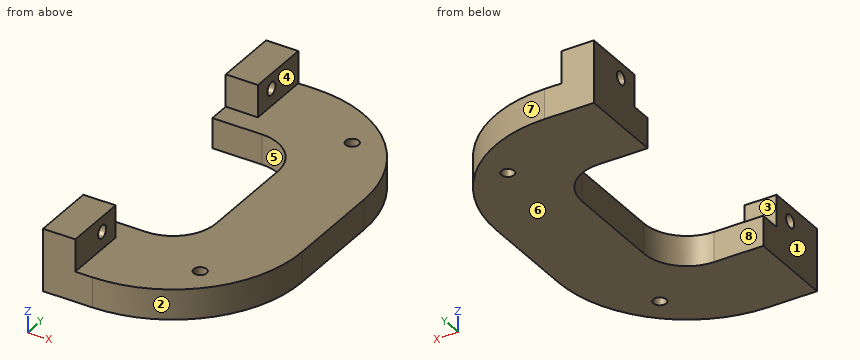
```python
from build123d import *

# Parameters (mm, degrees)
BOSS_EXTRUDE4_DEPTH = 7
SKETCH6_W           = 7.5
SKETCH6_H           = 20
BOSS_EXTRUDE5_DEPTH = 7.5
SKETCH7_R           = 1.5
CUT_EXTRUDE3_DEPTH  = 7.5
SKETCH8_R           = 1.5
CUT_EXTRUDE4_DEPTH  = 7.5
SKETCH9_W           = 7.5
SKETCH9_H           = 5
CUT_EXTRUDE5_DEPTH  = 7.5


with BuildPart() as part:
    # Sketch1 → Boss-Extrude4 (new body)
    with BuildSketch(Plane.XY):
        with BuildLine():
            Line((41.5, -11.5), (41.5, 11.5))
            ThreePointArc((41.5, 11.5), (32.713203436, 32.713203436), (11.5, 41.5))
            Line((11.5, 41.5), (0, 41.5))
            Line((0, 41.5), (0, 21.5))
            Line((0, 21.5), (11.5, 21.5))
            ThreePointArc((11.5, 21.5), (18.571067812, 18.571067812), (21.5, 11.5))
            Line((21.5, 11.5), (21.5, -11.5))
            ThreePointArc((21.5, -11.5), (18.571067812, -18.571067812), (11.5, -21.5))
            Line((11.5, -21.5), (0, -21.5))
            Line((0, -21.5), (0, -41.5))
            Line((0, -41.5), (11.5, -41.5))
            ThreePointArc((11.5, -41.5), (32.713203436, -32.713203436), (41.5, -11.5))
        make_face()
    extrude(amount=BOSS_EXTRUDE4_DEPTH)

    # Sketch6 → Boss-Extrude5 (add)
    with BuildSketch(Plane.XY.offset(7)):
        with Locations((3.75, 31.5)):
            Rectangle(SKETCH6_W, SKETCH6_H)
        with Locations((3.75, -31.5)):
            Rectangle(SKETCH6_W, SKETCH6_H)
    extrude(amount=BOSS_EXTRUDE5_DEPTH)

    # Sketch7 → Cut-Extrude3 (cut)
    with BuildSketch(Plane(origin=(7.5, 0, 0), x_dir=(0, 0, -1), z_dir=(1, 0, 0))):
        with Locations((-11, 31.5)):
            Circle(SKETCH7_R)
        with Locations((-11, -31.5)):
            Circle(SKETCH7_R)
    extrude(amount=-CUT_EXTRUDE3_DEPTH, mode=Mode.SUBTRACT)

    # Sketch8 → Cut-Extrude4 (cut)
    with BuildSketch(Plane.XY.offset(7)):
        with Locations((28.284271247, 28.284271247)):
            Circle(SKETCH8_R)
        with Locations((28.284271247, -28.284271247)):
            Circle(SKETCH8_R)
    extrude(amount=-CUT_EXTRUDE4_DEPTH, mode=Mode.SUBTRACT)

    # Sketch9 → Cut-Extrude5 (cut)
    with BuildSketch(Plane(origin=(7.5, 0, 0), x_dir=(0, 0, -1), z_dir=(1, 0, 0))):
        with Locations((-10.75, 24)):
            Rectangle(SKETCH9_W, SKETCH9_H)
        with Locations((-10.75, -24)):
            Rectangle(SKETCH9_W, SKETCH9_H)
    extrude(amount=-CUT_EXTRUDE5_DEPTH, mode=Mode.SUBTRACT)


solid = part.part
```
Could you check a few things on this model? Use its own coordinates, in mm. Face numbers are marked on the shaded views. A direction names the side the tool comes from. Round coordinates to 2 decimals unless told otherwise and drop trailing zeros. Write each loop counter-clockwise with the first axis right and the second up, starting at its lowest first coordinate (ties: lowest second). Pieces come first, ordered by that corner, then holes.
(1) Suppose I cut it at D-D on x = 37.5. Write out the boundary of the cut face in (y, z).
Findings below:
outline: (-26.47, 0) - (26.47, 0) - (26.47, 7) - (-26.47, 7) - close
(2) Thinking about a two-plate mould opening in Y: for the marked faces 6, 7 and 8, which applies, +Y half, -Y half, draft (parallel to the pull), parting line (faces both ways), or undercut?
Findings below:
face 6: draft
face 7: +Y half
face 8: undercut
(3) Suppose I cut it at A-A on z = 11. Write out the boundary of the cut face in (x, y).
Findings below:
outline: (0, -41.5) - (7.5, -41.5) - (7.5, -33) - (0, -33) - close; (0, -30) - (7.5, -30) - (7.5, -26.5) - (0, -26.5) - close; (0, 26.5) - (7.5, 26.5) - (7.5, 30) - (0, 30) - close; (0, 33) - (7.5, 33) - (7.5, 41.5) - (0, 41.5) - close
(4) For pin 1 (4 mm diameter, centred on y = -31.5, z = 11, fed in from -X); pin 2 (3.5 mm diameter, centred on y = -3.5, z = 4, fed in from -X); pin 3 (2 mm diameter, centred on y = 35.5, z = 11.5, fed in from +X); pin 4 (4 mm diameter, centred on x = 19, z = 6.5, fed in from -Y), each with a flat end and sliding along its axis, tell me the tip position at first contact or that it passes through.
Findings below:
pin 1: stops at x = 0
pin 2: stops at x = 21.5
pin 3: stops at x = 7.5
pin 4: stops at y = -40.99
(5) Which directions (+Z, -Z, +X, -X, +Y, -Y) give clear straight access to the entire face, cutting with the end or side of a thin tool? Please do the marked faces 1, 2, 3, 4 and 5.
Findings below:
face 1: +Z, -Z, -X, +Y, -Y
face 2: +Z, -Z, +X, -Y
face 3: +Z, +X, -X
face 4: +Z, +X, +Y, -Y
face 5: +Z, -Z, -X
(6) If I drill on probe 1 along Y at (x, z) = (5.25, 11); probe 2 along Y at (x, z) = (5, 1.5); probe 3 along Z at (x, y) = (24, -17), over which ranges is the centre line in solid material (lowest first)?
Findings below:
probe 1: y = -41.5 to -33, -30 to -26.5, 26.5 to 30, 33 to 41.5
probe 2: y = -41.5 to -21.5, 21.5 to 41.5
probe 3: z = 0 to 7
(7) Suppose I cut it at B-B on y = 31.5. Write out the boundary of the cut face in (x, z), and give its area (3 significant figures).
Findings below:
outline: (0, 0) - (33.86, 0) - (33.86, 7) - (7.5, 7) - (7.5, 9.5) - (0, 9.5) - close; (0, 12.5) - (7.5, 12.5) - (7.5, 14.5) - (0, 14.5) - close
area: 271 mm2
(8) Suppose I cut it at C-C on z = 3. Write out the boundary of the cut face in (x, y).
Findings below:
outline: (0, -41.5) - (11.5, -41.5) arc R30 ccw to (41.5, -11.5) - (41.5, 11.5) arc R30 ccw to (11.5, 41.5) - (0, 41.5) - (0, 21.5) - (11.5, 21.5) arc R10 cw to (21.5, 11.5) - (21.5, -11.5) arc R10 cw to (11.5, -21.5) - (0, -21.5) - close; hole circle Ø3 at (28.28, -28.28); hole circle Ø3 at (28.28, 28.28)
